Design review of the part built by this model. Coordinates are the model's own, in mm. A direction names the side the tool comes from. Round coordinates to 2 decimals unless told otherwise and drop trailing zeros. Write each loop counter-clockwise with the first axis right and the second up, starting at its lowest first coordinate (ties: lowest second). Pieces come first, ordered by that corner, then holes. Notation, with made-up numbers: (59.25, 65) - (81.25, 65) arc R3 ccw to (81.25, 70) - close; hole circle Ø5 at (52, -31). An arc over 180 degrees is marked (long way). Use one line per item in the form item = value.
```python
from build123d import *

# Parameters (mm, degrees)
SKETCH1_W               = 216
SKETCH1_H               = 30
BOSS_EXTRUDE1_DEPTH     = 15
CUT_EXTRUDE1_REACH      = 220.589
SKETCH2_W               = 35
SKETCH2_H               = 15
SKETCH2_H_2             = 7.5
FILLET1_R               = 15
CUT_EXTRUDE2_DEPTH      = 221.127235934
CUT_EXTRUDE2_DEPTH_BACK = 221.127235934
SKETCH3_R               = 5
FILLET3_R               = 15


with BuildPart() as part:
    # Sketch1 → Boss-Extrude1 (new, symmetric)
    with BuildSketch(Plane.XY):
        with Locations((108, 15)):
            Rectangle(SKETCH1_W, SKETCH1_H)
    extrude(amount=BOSS_EXTRUDE1_DEPTH, both=True)

    # Sketch2 → Cut-Extrude1 (cut, up to next)
    with BuildSketch(Plane(origin=(0, 30, 0), x_dir=(1, 0, 0), z_dir=(0, 1, 0)), mode=Mode.PRIVATE) as cut_extrude1_sk1:
        with Locations((17.5, 0)):
            Rectangle(SKETCH2_W, SKETCH2_H)
    cut_extrude1_tool1 = extrude(cut_extrude1_sk1.sketch, amount=-CUT_EXTRUDE1_REACH, mode=Mode.PRIVATE) & part.part
    # Sketch2 → Cut-Extrude1 (cut, up to next)
    with BuildSketch(Plane(origin=(0, 30, 0), x_dir=(1, 0, 0), z_dir=(0, 1, 0)), mode=Mode.PRIVATE) as cut_extrude1_sk2:
        with Locations((198.5, 11.25)):
            Rectangle(SKETCH2_W, SKETCH2_H_2)
    cut_extrude1_tool2 = extrude(cut_extrude1_sk2.sketch, amount=-CUT_EXTRUDE1_REACH, mode=Mode.PRIVATE) & part.part
    # Sketch2 → Cut-Extrude1 (cut, up to next)
    with BuildSketch(Plane(origin=(0, 30, 0), x_dir=(1, 0, 0), z_dir=(0, 1, 0)), mode=Mode.PRIVATE) as cut_extrude1_sk3:
        with Locations((198.5, -11.25)):
            Rectangle(SKETCH2_W, SKETCH2_H_2)
    cut_extrude1_tool3 = extrude(cut_extrude1_sk3.sketch, amount=-CUT_EXTRUDE1_REACH, mode=Mode.PRIVATE) & part.part
    add(cut_extrude1_tool1.solids().sort_by_distance((17.5, 30, 0))[0], mode=Mode.SUBTRACT)
    add(cut_extrude1_tool2.solids().sort_by_distance((198.5, 30, -11.25))[0], mode=Mode.SUBTRACT)
    add(cut_extrude1_tool3.solids().sort_by_distance((198.5, 30, 11.25))[0], mode=Mode.SUBTRACT)

    # Fillet1
    fillet1_edges = [part.edges().sort_by_distance(p)[0] for p in [
        (216, 0, 0),
        (216, 30, 0),
        (0, 0, 11.25),
        (0, 0, -11.25),
        (0, 30, -11.25),
        (0, 30, 11.25),
    ]]
    fillet(fillet1_edges, radius=FILLET1_R - 0.0001)  # a hair under: the kernel refuses the full size

    # Sketch3 → Cut-Extrude2 (cut, two sides: drawn at the far end of the back side and taken through both)
    with BuildSketch(Plane.XY.offset(15).offset(-CUT_EXTRUDE2_DEPTH_BACK)):
        with Locations((15, 15)):
            Circle(SKETCH3_R)
        with Locations((201, 15)):
            Circle(SKETCH3_R)
    extrude(amount=CUT_EXTRUDE2_DEPTH + CUT_EXTRUDE2_DEPTH_BACK, mode=Mode.SUBTRACT)

    # Fillet3
    fillet3_edges = [part.edges().sort_by_distance(p)[0] for p in [
        (181, 0, -11.25),
        (181, 30, -11.25),
        (181, 0, 11.25),
        (181, 30, 11.25),
    ]]
    fillet(fillet3_edges, radius=FILLET3_R - 0.0001)  # a hair under: the kernel refuses the full size


solid = part.part
```
Q1. To check wall thickness, follow line 1 along X through (y, z) = (15, 12.25); line 2 along Y through (x, z) = (15, -11.25); line 3 along Z through (x, y) = (17.5, 8). State the ranges of each line that lie inside material, in increasing order. Write a range as from..to.
Calculated:
line_1 = 0..10, 20..181
line_2 = 0..10, 20..30
line_3 = -15..-7.5, 7.5..15
Q2. For P1, Ø3, axis at y = 21, z = -8.5, coming from the -X side; P2, Ø13, axis at x = 201, y = 15, coming from the +Z side; P3, Ø8, axis at y = 20.5, z = -1.5, coming from the +X side, all flat-tipped, find the tip position at first contact; note any pin that passes through.
Calculated:
P1 = 0.69
P2 = 7.5
P3 = 215.92
Q3. Machinability: for faces 5 (the cylindrical face through (176.49, 25.72, 11.2)), 6 (the flat face through (21, 15, -7.5)), 7 (the cylindrical face through (203.307, 10.564, -0.105)), 8 (the cylindrical face through (176.49, 25.72, -11.3)), 9 (the cylindrical face through (176.49, 4.28, -11.3)), which of the approach directions +Z, -Z, +X, -X, +Y, -Y give a long, thin tool a straight path to every point of the face, cutting with its end or side? Answer none if there is none.
Calculated:
face_5 = +Z, +X, +Y
face_6 = -X, +Y, -Y
face_7 = +Z, -Z
face_8 = -Z, +X, +Y
face_9 = -Z, +X, -Y
Q4. Draft analysis for pull direction Z (two halves, no side actions). For faces 1 (the flat face through (89, 15, 15)), 2 (the cylindrical face through (4.28, 25.49, -11.3)), 3 (the flat face through (21, 15, 7.5)), 4 (the flat face through (35, 15, 0)), state which applies: released by +Z, released by -Z, zero draft, split by the parting line, or undercut.
Calculated:
face_1 = released by +Z
face_2 = zero draft
face_3 = undercut
face_4 = undercut
Q5. We need section C-C on y = 3. Write out the cut boundary in (x, z), then the cut area to 3 significant figures.
Calculated:
outline = (6, -15) - (175, -15) - (175, -7.5) - (210, -7.5) - (210, 7.5) - (175, 7.5) - (175, 15) - (6, 15) - (6, 7.5) - (35, 7.5) - (35, -7.5) - (6, -7.5) - close
area = 5,160 mm2
Q6. We need section B-B on y = 12. Write out the cut boundary in (x, z), then the cut area to 3 significant figures.
Calculated:
outline = (0.3, -15) - (11, -15) - (11, -7.5) - (0.3, -7.5) - close; (0.3, 7.5) - (11, 7.5) - (11, 15) - (0.3, 15) - close; (19, -15) - (180.7, -15) - (180.7, -7.5) - (197, -7.5) - (197, 7.5) - (180.7, 7.5) - (180.7, 15) - (19, 15) - (19, 7.5) - (35, 7.5) - (35, -7.5) - (19, -7.5) - close; (205, -7.5) - (215.7, -7.5) - (215.7, 7.5) - (205, 7.5) - close
area = 5,180 mm2
